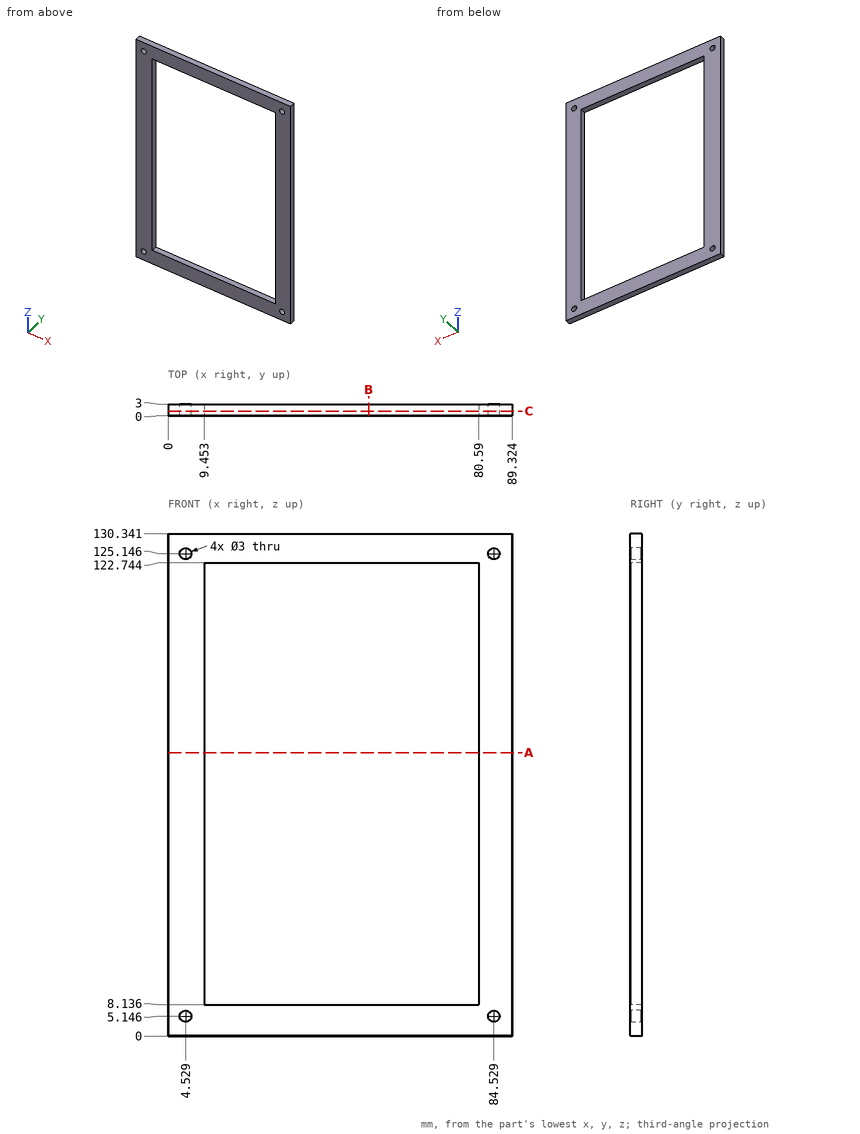
Could you check a few things on this drawing? It's one solid part, dimensions in mm from its lowest x, y, z. Give positions to 0.01 mm unless a question says otherwise; leave off trailing zeros. Order: outer loops, then holes, each group sorted by start corner. A loop starts at its lowest first (then second) coordinate and runs counter-clockwise, first axis right, second up. Notation, with made-up numbers: (-13, 49.5) -> (45, 49.5) arc R23 cw to (45, 57.5) -> close; hole circle Ø6 at (18.5, 83). An arc over 180 degrees is marked (long way). Answer in a Markdown table with one row per item. Add a question column.
Item 1: Imagine slicing it at B-B (x = 52). List the corners of the cut face in (y, z) for me (1 decimal), and give its area (3 significant figures).
Item 2: Please list where these lines run through material, in increasing order: probe 1 along Z at (x, y) = (68, 2) (1 decimal); probe 2 along X at (y, z) = (1, 58) (1 decimal).
Item 3: I'm going to push a flat-ended pin straight in: P1, Ø3.5, axis at x = 84.53, z = 125.15, coming from the -Y side. Where does the tip first touch, or does it pass through?
Item 4: Imagine slicing it at A-A (z = 73.5). List the corners of the cut face in (x, y) for me (1 decimal).
Item 5: Imagine slicing it at C-C (y = 1.15). List the corners of the cut face in (x, z) for me (1 decimal), and give its area (3 significant figures).
Result:
| question | item | result |
|---|---|---|
| 1 | outline | (0, 0) -> (3, 0) -> (3, 8.1) -> (0, 8.1) -> close; (0, 122.7) -> (3, 122.7) -> (3, 130.3) -> (0, 130.3) -> close |
| 1 | area | 47.2 mm2 |
| 2 | probe 1 | 0 to 8.1, 122.7 to 130.3 |
| 2 | probe 2 | 0 to 9.5, 80.6 to 89.3 |
| 3 | P1 | y = 0 |
| 4 | outline | (0, 0) -> (9.5, 0) -> (9.5, 3) -> (0, 3) -> close; (80.6, 0) -> (89.3, 0) -> (89.3, 3) -> (80.6, 3) -> close |
| 5 | outline | (0, 0) -> (89.3, 0) -> (89.3, 130.3) -> (0, 130.3) -> close; hole circle Ø3 at (4.5, 5.1); hole circle Ø3 at (4.5, 125.1); hole (9.5, 8.1) -> (80.6, 8.1) -> (80.6, 122.7) -> (9.5, 122.7) -> close; hole circle Ø3 at (84.5, 5.1); hole circle Ø3 at (84.5, 125.1) |
| 5 | area | 3,460 mm2 |
